Part model, mm, in its own coordinate system. Face numbers are marked on the shaded views. Give positions to 0.01 mm unless a question says otherwise; leave off trailing zeros. Order: outer loops, then holes, each group sorted by start corner. A loop starts at its lowest first (then second) coordinate and runs counter-clockwise, first axis right, second up. Notation, with made-up numbers: M 58,18.25 L 112,18.25 A12 cw 112,35.25 Z; hole C 80,32 d3. An arc over 180 degrees is marked long. Answer as a JSON object with one key per item and string values.
from build123d import *

# Parameters (mm, degrees)
SKETCH_1_W      = 71
SKETCH_1_H      = 47
SKETCH_1_R      = 11
SKETCH_1_R_2    = 3.5
EXTRUDE_2_DEPTH = 5
FILLET_1_R      = 8


with BuildPart() as part:
    # 草图1 → 凸台-拉伸2 (new body)
    with BuildSketch(Plane.XY):
        Rectangle(SKETCH_1_W, SKETCH_1_H)
        with Locations((-23, 11.5)):
            Circle(SKETCH_1_R, mode=Mode.SUBTRACT)
        with Locations((0, 11.5)):
            Circle(SKETCH_1_R, mode=Mode.SUBTRACT)
        with Locations((23, 11.5)):
            Circle(SKETCH_1_R, mode=Mode.SUBTRACT)
        with Locations((23, -11.5)):
            Circle(SKETCH_1_R, mode=Mode.SUBTRACT)
        with Locations((0, -11.5)):
            Circle(SKETCH_1_R, mode=Mode.SUBTRACT)
        with Locations((-23, -11.5)):
            Circle(SKETCH_1_R, mode=Mode.SUBTRACT)
        with Locations((11.5, 0)):
            Circle(SKETCH_1_R_2, mode=Mode.SUBTRACT)
        with Locations((-11.5, 0)):
            Circle(SKETCH_1_R_2, mode=Mode.SUBTRACT)
    extrude(amount=-EXTRUDE_2_DEPTH)

    # 圆角1
    fillet_1_edges = [part.edges().sort_by_distance(p)[0] for p in [
        (35.5, -23.5, -2.5),
        (-35.5, -23.5, -2.5),
        (-35.5, 23.5, -2.5),
        (35.5, 23.5, -2.5),
    ]]
    fillet(fillet_1_edges, radius=FILLET_1_R)


solid = part.part
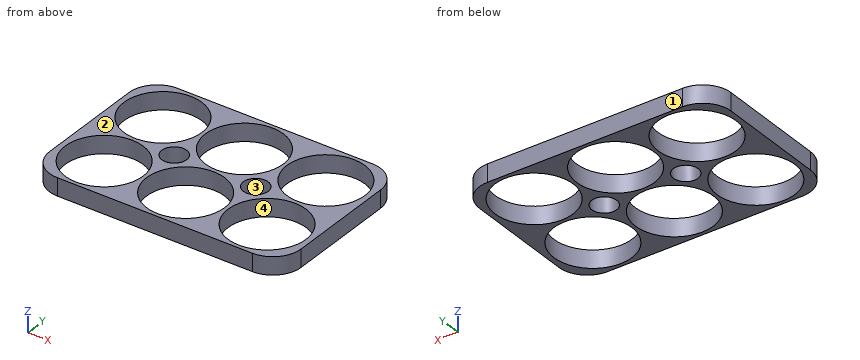
1. Cut at A-A on x = -23. Give the cut face in (y, z), plus the area to 3 significant figures.
Worked answers:
{"outline": "M -23.5,-5 L -22.5,-5 L -22.5,0 L -23.5,0 Z; M -0.5,-5 L 0.5,-5 L 0.5,0 L -0.5,0 Z; M 22.5,-5 L 23.5,-5 L 23.5,0 L 22.5,0 Z", "area": "15.0 mm^2"}
2. Cut at D-D on x = -10. Give the cut face in (y, z), plus the area to 3 significant figures.
Worked answers:
{"outline": "M -23.5,-5 L -16.08,-5 L -16.08,0 L -23.5,0 Z; M -6.92,-5 L -3.16,-5 L -3.16,0 L -6.92,0 Z; M 3.16,-5 L 6.92,-5 L 6.92,0 L 3.16,0 Z; M 16.08,-5 L 23.5,-5 L 23.5,0 L 16.08,0 Z", "area": "112 mm^2"}
3. Two-plate mould, pull along Y, no slides. Class the marked faces 1, 2, 3 and 4: +Y half, -Y half, draft (parallel to the pull), parting line (faces both ways), or undercut.
Worked answers:
{"face 1": "+Y half", "face 2": "draft", "face 3": "undercut", "face 4": "undercut"}
4. Cut at C-C on z = -2.6. State how many separate pieces and enclosed holes the cut face has, plus the area to 3 significant figures.
Worked answers:
{"separate pieces": "1", "enclosed holes": "8", "area": "924 mm^2"}
5. Pin check, flat tips, straight feed: P1, Ø13, axis at x = 23, y = -11.5, coming from the -Z side; P2, Ø1, axis at y = -17.5, z = -2.5, coming from the -X side. Stop position of each tip, or through.
Worked answers:
{"P1": "passes through", "P2": "stops at x = -35.36"}
6. Probe line 1 along Y through (x, z) = (23, -2.4); line 2 along Y through (x, z) = (11.5, -1.55); line 3 along Y through (x, z) = (-24.5, -3.05). List the from-to ranges inside material, lowest first.
Worked answers:
{"line 1": "y = -23.5 to -22.5, -0.5 to 0.5, 22.5 to 23.5", "line 2": "y = -23.5 to -3.5, 3.5 to 23.5", "line 3": "y = -23.5 to -22.4, -0.6 to 0.6, 22.4 to 23.5"}
7. Cut at B-B on y = -11.5. Give the cut face in (x, z), plus the area to 3 significant figures.
Worked answers:
{"outline": "M -35.5,-5 L -34,-5 L -34,0 L -35.5,0 Z; M -12,-5 L -11,-5 L -11,0 L -12,0 Z; M 11,-5 L 12,-5 L 12,0 L 11,0 Z; M 34,-5 L 35.5,-5 L 35.5,0 L 34,0 Z", "area": "25.0 mm^2"}
